Answer from the drawing. Dimensions are ordinates in mm from the lowest x, y and z of the part. A direction names the side the tool comes from. Round coordinates to 2 decimals unless told otherwise and drop trailing zeros. Write each loop counter-clockwise with the first axis right and the second up, starting at its lowest first coordinate (ties: lowest second). Pieces come first, ordered by that corner, then holes. Notation, with made-up numbers: (57.5, -16.75) - (107.5, -16.75) arc R19 ccw to (107.5, 11.25) - close; hole circle Ø1 at (67.25, 31.5). An arc over 180 degrees is marked (long way). Use a Markdown table: item, result. Add a question column.
1) A cutting plane is placed at D-D (z = 1.15). Give the vertices of the cut face in (x, y), then the cut area to 3 significant figures.
2) A cutting plane is placed at B-B (x = 10.25). Give the vertices of the cut face in (y, z).
3) Find the intervals of material crossed by probe 1 along X at (y, z) = (12, 1.8); probe 2 along Y at (x, z) = (12.25, 2); probe 3 along Y at (x, z) = (4.5, 0.95), in increasing order. Write a range as from..to.
4) A tool of negligible diameter and unlimited length cuts with its end or side. For the marked faces 4 and 5, from which of +Z, -Z, +X, -X, +Y, -Y can it reach the whole face along a straight path? Write none if from no direction.
5) Determine the mould class of the marked faces 1, 2 and 3 for opening direction X: +X half, -X half, draft (parallel to the pull), parting line (faces both ways), or undercut.
6) A cutting plane is placed at A-A (y = 17.5). Give the vertices of the cut face in (x, z).
7) This flat-tipped pin is pushed along its axis until it touches: P1, Ø3, axis at x = 4.5, y = 17.5, coming from the +Z side. Where does it stop, or does it pass through?
8) A cutting plane is placed at C-C (y = 13.5). Give the vertices of the cut face in (x, z).
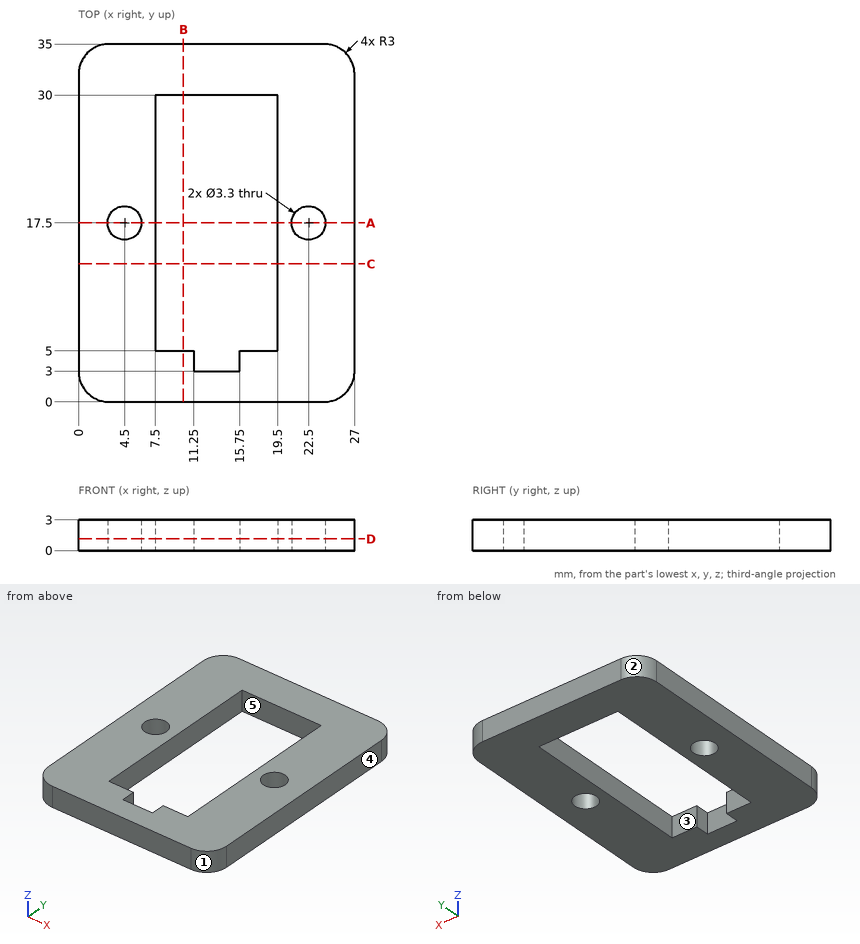
Entries:
| question | item | result |
|---|---|---|
| 1 | outline | (0, 3) arc R3 ccw to (3, 0) - (24, 0) arc R3 ccw to (27, 3) - (27, 32) arc R3 ccw to (24, 35) - (3, 35) arc R3 ccw to (0, 32) - close; hole circle Ø3.3 at (4.5, 17.5); hole (7.5, 5) - (11.25, 5) - (11.25, 3) - (15.75, 3) - (15.75, 5) - (19.5, 5) - (19.5, 30) - (7.5, 30) - close; hole circle Ø3.3 at (22.5, 17.5) |
| 1 | area | 611 mm² |
| 2 | outline | (0, 0) - (5, 0) - (5, 3) - (0, 3) - close; (30, 0) - (35, 0) - (35, 3) - (30, 3) - close |
| 3 | probe 1 | x = 0..7.5, 19.5..27 |
| 3 | probe 2 | y = 0..3, 30..35 |
| 3 | probe 3 | y = 0..15.85, 19.15..35 |
| 4 | face 4 | +Z, -Z, +X, +Y, -Y |
| 4 | face 5 | +Z, -Z |
| 5 | face 1 | +X half |
| 5 | face 2 | -X half |
| 5 | face 3 | undercut |
| 6 | outline | (0, 0) - (2.85, 0) - (2.85, 3) - (0, 3) - close; (6.15, 0) - (7.5, 0) - (7.5, 3) - (6.15, 3) - close; (19.5, 0) - (20.85, 0) - (20.85, 3) - (19.5, 3) - close; (24.15, 0) - (27, 0) - (27, 3) - (24.15, 3) - close |
| 7 | P1 | passes through |
| 8 | outline | (0, 0) - (7.5, 0) - (7.5, 3) - (0, 3) - close; (19.5, 0) - (27, 0) - (27, 3) - (19.5, 3) - close |
